Geometry check sheet. Reference: drawing and pictorial views, mm from the part's lowest x, y, z. A direction names the side the tool comes from. Give positions to 0.01 mm unless a question says otherwise; leave off trailing zeros. Order: outer loops, then holes, each group sorted by start corner. A loop starts at its lowest first (then second) coordinate and runs counter-clockwise, first axis right, second up.
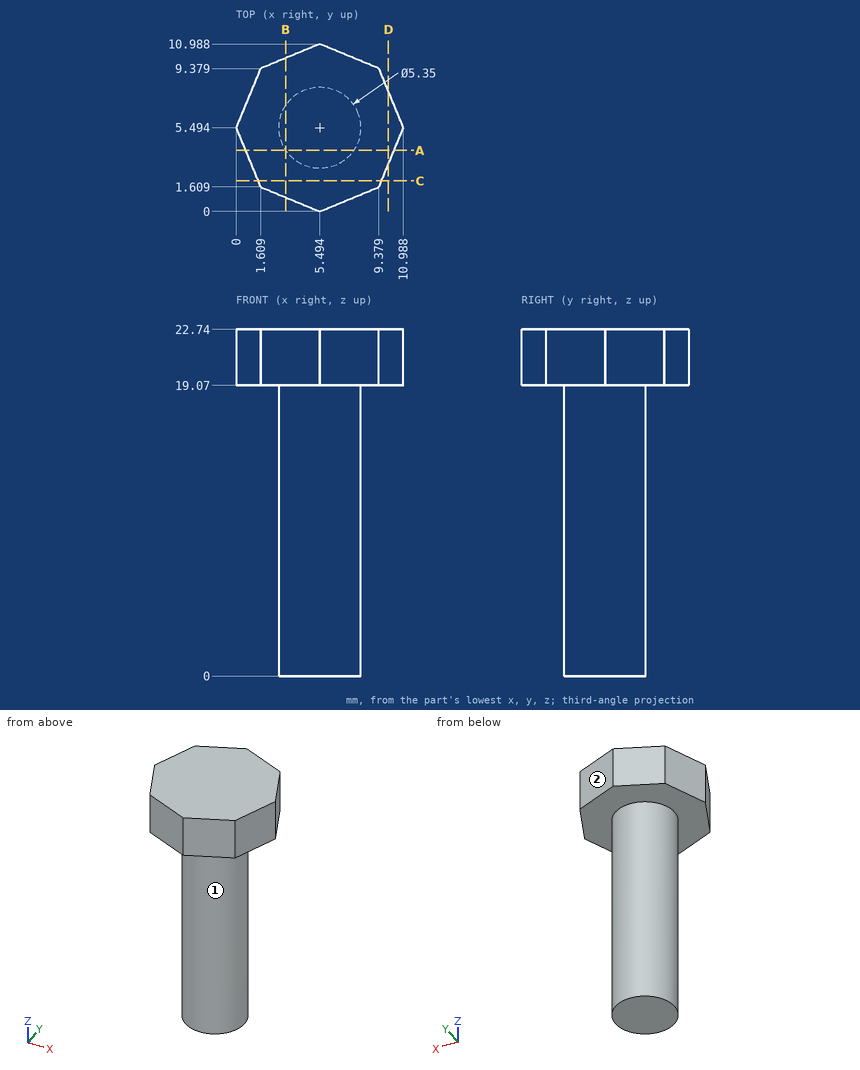
(1) Sectioned sample at B-B (x = 3.25). Enter the section's corners in (y, z).
(2) Go/stop test with flat-tipped pins: P1, Ø6, axis at x = 5.5, z = 2.5, coming from the -Y side; P2, Ø2, axis at y = 5.5, z = 2.5, coming from the +X side; P3, Ø6, axis at x = 1.5, z = 13.5, coming from the -Y side. Record where each tip stops, or that it passes through.
(3) Sectioned sample at A-A (y = 4). Enter the section's corners in (x, z) (1 decimal).
(4) Sectioned sample at D-D (x = 10). Enter the section's corners in (y, z).
(5) Sectioned sample at C-C (y = 2). Enter the section's corners in (x, z), plus the area to 3 significant figures.
(6) Thickness scan on L1, parallel to Z at x = 2.5, y = 5.5; L2, parallel to Y at x = 5.5, z = 21.75 (1 decimal); L3, parallel to Y at x = 5.5, z = 2. Record the ranges inside material, lowest first.
(7) Tool access check on the marked faces 1 and 2. Record the directions out of +Z, -Z, +X, -X, +Y, -Y that give a thin tool (end or side, any length) a straight path to the whole face; none if there is none.
Values follow:
1. outline: (0.93, 19.07) - (4.04, 19.07) - (4.04, 0) - (6.95, 0) - (6.95, 19.07) - (10.06, 19.07) - (10.06, 22.74) - (0.93, 22.74) - close
2. P1: stops at y = 2.82
2. P2: stops at x = 8.17
2. P3: stops at y = 3.01
3. outline: (0.6, 19.1) - (3.3, 19.1) - (3.3, 0) - (7.7, 0) - (7.7, 19.1) - (10.4, 19.1) - (10.4, 22.7) - (0.6, 22.7) - close
4. outline: (3.11, 19.07) - (7.88, 19.07) - (7.88, 22.74) - (3.11, 22.74) - close
5. outline: (1.45, 19.07) - (9.54, 19.07) - (9.54, 22.74) - (1.45, 22.74) - close
5. area: 29.7 mm2
6. L1: z = 19.07 to 22.74
6. L2: y = 0 to 11
6. L3: y = 2.82 to 8.17
7. face 1: -Z
7. face 2: +Z, -Z, +X, +Y
